from build123d import *

# Parameters (mm, degrees)
F3_DEPTH  = 6.86
F4_SIZE   = 0.13
F5_SIZE   = 0.06
F6_SIZE   = 0.03
F8_DEPTH  = 6.79
F10_DEPTH = 14.1


with BuildPart() as f1:
    # F0 (on Top) → F1 (revolve)
    with BuildSketch(Plane.XY):
        Polygon((-33.448007, 1.065), (-29.198007, 1.065), (-29.198007, 1.27955), (-29.778007, 1.27955), (-29.778007, 1.5), (-30.008007, 1.5), (-30.008007, 2.5), (-30.138007, 2.5), (-30.138007, 2.375), (-32.138007, 2.375), (-32.138007, 2.5), (-32.268007, 2.5), (-32.268007, 1.5), (-32.491007, 1.5), (-32.491007, 1.27955), (-33.111007, 1.27955), (-33.111007, 1.215), (-34.191007, 1.215), (-34.191007, 0), (-33.448007, 0), align=None)
    revolve(axis=Axis((-33.819507, 0, 0), (1, 0, 0)))

    # F2 (on face) → F3 (cut)
    with BuildSketch(Plane(origin=(-34.191007, 0, 0), x_dir=(0, -1, 0), z_dir=(-1, 0, 0))):
        with BuildLine():
            Line((-0.07875, 0.268), (-0.07875, 0.180575))
            ThreePointArc((-0.07875, 0.180575), (0, -0.197), (0.07875, 0.180575))
            Line((0.07875, 0.180575), (0.07875, 0.268))
            Line((0.07875, 0.268), (0, 0.268))
            Line((0, 0.268), (-0.07875, 0.268))
        make_face()
    extrude(amount=-F3_DEPTH, mode=Mode.SUBTRACT)

    # F4
    f4_edges = [f1.edges().sort_by_distance(p)[0] for p in [
        (-34.191007, -1.215, 0),
        (-32.491007, -1.5, 0),
        (-29.778007, -1.5, 0),
    ]]
    chamfer(f4_edges, length=F4_SIZE)

    # F5
    f5_edges = [f1.edges().sort_by_distance(p)[0] for p in [
        (-29.198007, -1.27955, 0),
    ]]
    chamfer(f5_edges, length=F5_SIZE)

    # F6
    f6_edges = [f1.edges().sort_by_distance(p)[0] for p in [
        (-33.111007, -1.27955, 0),
    ]]
    chamfer(f6_edges, length=F6_SIZE)

    # F7 (on face) → F8 (cut)
    with BuildSketch(Plane(origin=(-32.268007, 0, 0), x_dir=(0, -1, 0), z_dir=(-1, 0, 0))):
        with BuildLine():
            ThreePointArc((-0.503698, 1.550222), (0, 1.63), (0.503698, 1.550222))
            ThreePointArc((0.503698, 1.550222), (0.856518, 1.729993), (0.676747, 2.082814))
            ThreePointArc((0.676747, 2.082814), (0, 2.19), (-0.676747, 2.082814))
            ThreePointArc((-0.676747, 2.082814), (-0.856518, 1.729993), (-0.503698, 1.550222))
        make_face()
        with BuildLine():
            ThreePointArc((-1.594381, 0.338896), (-1.411621, 0.815), (-1.090683, 1.211326))
            ThreePointArc((-1.090683, 1.211326), (-1.069959, 1.606763), (-1.465396, 1.627487))
            ThreePointArc((-1.465396, 1.627487), (-1.896596, 1.095), (-2.142143, 0.455327))
            ThreePointArc((-2.142143, 0.455327), (-1.926477, 0.12323), (-1.594381, 0.338896))
        make_face()
        with BuildLine():
            ThreePointArc((-1.090683, -1.211326), (-1.411621, -0.815), (-1.594381, -0.338896))
            ThreePointArc((-1.594381, -0.338896), (-1.926477, -0.12323), (-2.142143, -0.455327))
            ThreePointArc((-2.142143, -0.455327), (-1.896596, -1.095), (-1.465396, -1.627487))
            ThreePointArc((-1.465396, -1.627487), (-1.069959, -1.606763), (-1.090683, -1.211326))
        make_face()
        with BuildLine():
            ThreePointArc((0.503698, -1.550222), (0, -1.63), (-0.503698, -1.550222))
            ThreePointArc((-0.503698, -1.550222), (-0.856518, -1.729993), (-0.676747, -2.082814))
            ThreePointArc((-0.676747, -2.082814), (0, -2.19), (0.676747, -2.082814))
            ThreePointArc((0.676747, -2.082814), (0.856518, -1.729993), (0.503698, -1.550222))
        make_face()
        with BuildLine():
            ThreePointArc((1.594381, -0.338896), (1.411621, -0.815), (1.090683, -1.211326))
            ThreePointArc((1.090683, -1.211326), (1.069959, -1.606763), (1.465396, -1.627487))
            ThreePointArc((1.465396, -1.627487), (1.896596, -1.095), (2.142143, -0.455327))
            ThreePointArc((2.142143, -0.455327), (1.926477, -0.12323), (1.594381, -0.338896))
        make_face()
        with BuildLine():
            ThreePointArc((1.090683, 1.211326), (1.411621, 0.815), (1.594381, 0.338896))
            ThreePointArc((1.594381, 0.338896), (1.926477, 0.12323), (2.142143, 0.455327))
            ThreePointArc((2.142143, 0.455327), (1.896596, 1.095), (1.465396, 1.627487))
            ThreePointArc((1.465396, 1.627487), (1.069959, 1.606763), (1.090683, 1.211326))
        make_face()
    extrude(amount=-F8_DEPTH, mode=Mode.SUBTRACT)

    # F9 (on face) → F10 (cut)
    with BuildSketch(Plane(origin=(-32.268007, 0, 0), x_dir=(0, -1, 0), z_dir=(-1, 0, 0))):
        with BuildLine():
            ThreePointArc((-1.594381, 0.338896), (-1.411621, 0.815), (-1.090683, 1.211326))
            ThreePointArc((-1.090683, 1.211326), (-1.069959, 1.606763), (-1.465396, 1.627487))
            ThreePointArc((-1.465396, 1.627487), (-1.896596, 1.095), (-2.142143, 0.455327))
            ThreePointArc((-2.142143, 0.455327), (-1.926477, 0.12323), (-1.594381, 0.338896))
        make_face()
        with BuildLine():
            ThreePointArc((-2.142143, -0.455327), (-1.896596, -1.095), (-1.465396, -1.627487))
            ThreePointArc((-1.465396, -1.627487), (-1.069959, -1.606763), (-1.090683, -1.211326))
            ThreePointArc((-1.090683, -1.211326), (-1.411621, -0.815), (-1.594381, -0.338896))
            ThreePointArc((-1.594381, -0.338896), (-1.926477, -0.12323), (-2.142143, -0.455327))
        make_face()
        with BuildLine():
            ThreePointArc((-0.676747, -2.082814), (0, -2.19), (0.676747, -2.082814))
            ThreePointArc((0.676747, -2.082814), (0.856518, -1.729993), (0.503698, -1.550222))
            ThreePointArc((0.503698, -1.550222), (0, -1.63), (-0.503698, -1.550222))
            ThreePointArc((-0.503698, -1.550222), (-0.856518, -1.729993), (-0.676747, -2.082814))
        make_face()
        with BuildLine():
            ThreePointArc((1.465396, -1.627487), (1.896596, -1.095), (2.142143, -0.455327))
            ThreePointArc((2.142143, -0.455327), (1.926477, -0.12323), (1.594381, -0.338896))
            ThreePointArc((1.594381, -0.338896), (1.411621, -0.815), (1.090683, -1.211326))
            ThreePointArc((1.090683, -1.211326), (1.069959, -1.606763), (1.465396, -1.627487))
        make_face()
        with BuildLine():
            ThreePointArc((2.142143, 0.455327), (1.896596, 1.095), (1.465396, 1.627487))
            ThreePointArc((1.465396, 1.627487), (1.069959, 1.606763), (1.090683, 1.211326))
            ThreePointArc((1.090683, 1.211326), (1.411621, 0.815), (1.594381, 0.338896))
            ThreePointArc((1.594381, 0.338896), (1.926477, 0.12323), (2.142143, 0.455327))
        make_face()
        with BuildLine():
            ThreePointArc((-0.503698, 1.550222), (0, 1.63), (0.503698, 1.550222))
            ThreePointArc((0.503698, 1.550222), (0.856518, 1.729993), (0.676747, 2.082814))
            ThreePointArc((0.676747, 2.082814), (0, 2.19), (-0.676747, 2.082814))
            ThreePointArc((-0.676747, 2.082814), (-0.856518, 1.729993), (-0.503698, 1.550222))
        make_face()
    extrude(amount=-F10_DEPTH, mode=Mode.SUBTRACT)


solid = f1.part
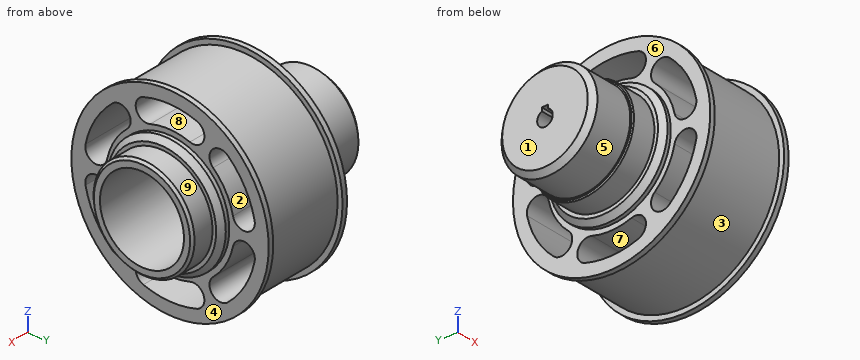
Could you check a few things on this model? Use its own coordinates, in mm. Face numbers are marked on the shaded views. A direction names the side the tool comes from. Give positions to 0.01 mm unless a question says otherwise; leave off trailing zeros. Loops run counter-clockwise (first coordinate to the right, second up) from the corner with the lowest first, then second, coordinate; pieces in that order, holes last. Notation, with made-up numbers: (54, 69.5) -> (83, 69.5) arc R31 cw to (83, 105.5) -> close; hole circle Ø10 at (24.5, -3.75). An arc over 180 degrees is marked (long way). Return JSON: item names as keys, results as strings.
Item 1: I'm going to push flat-ended pins straight in: pin 1 (2.5 mm diameter, centred on y = -1, z = -1, fed in from +X); pin 2 (1.7 mm diameter, centred on y = 0, z = 0, fed in from +X); pin 3 (2 mm diameter, centred on x = -30, z = -1.5, fed in from +Y). Where does each tip first touch, or does it pass through?
Geometry results:
{"pin 1": "stops at x = -29.2", "pin 2": "stops at x = -33.45", "pin 3": "stops at y = 2.45"}
Item 2: We'd pull the mould along Y, two halves only. Please class the marked faces 6, 7, 8 and 9: +Y half, -Y half, draft (parallel to the pull), parting line (faces both ways), or undercut.
Geometry results:
{"face 6": "draft", "face 7": "undercut", "face 8": "undercut", "face 9": "parting line"}
Item 3: If we section it at A-A on y = 1.8: List the corners of the cut face in (x, z) for me.
Geometry results:
{"outline": "(-32.27, -1.73) -> (-32.14, -1.73) -> (-32.14, -1.55) -> (-30.14, -1.55) -> (-30.14, -1.73) -> (-30.01, -1.73) -> (-30.01, -1.25) -> (-32.27, -1.25) -> close; (-32.27, -0.13) -> (-30.01, -0.13) -> (-30.01, 0.13) -> (-32.27, 0.13) -> close; (-32.27, 1.25) -> (-30.01, 1.25) -> (-30.01, 1.73) -> (-30.14, 1.73) -> (-30.14, 1.55) -> (-32.14, 1.55) -> (-32.14, 1.73) -> (-32.27, 1.73) -> close"}
Item 4: If we section it at B-B on x = -30.5: List the corners of the cut face in (y, z) for me (3 decimals), plus the area to 3 significant figures.
Geometry results:
{"outline": "circle Ø4.75 at (0, 0); hole (-2.142, -0.455) arc R2.19 ccw to (-1.465, -1.627) arc R0.28 ccw to (-1.091, -1.211) arc R1.63 cw to (-1.594, -0.339) arc R0.28 ccw to start; hole (-2.142, 0.455) arc R0.28 ccw to (-1.594, 0.339) arc R1.63 cw to (-1.091, 1.211) arc R0.28 ccw to (-1.465, 1.627) arc R2.19 ccw to start; hole circle Ø2.13 at (0, 0); hole (-0.677, -2.083) arc R2.19 ccw to (0.677, -2.083) arc R0.28 ccw to (0.504, -1.55) arc R1.63 cw to (-0.504, -1.55) arc R0.28 ccw to start; hole (-0.677, 2.083) arc R0.28 ccw to (-0.504, 1.55) arc R1.63 cw to (0.504, 1.55) arc R0.28 ccw to (0.677, 2.083) arc R2.19 ccw to start; hole (1.091, -1.211) arc R0.28 ccw to (1.465, -1.627) arc R2.19 ccw to (2.142, -0.455) arc R0.28 ccw to (1.594, -0.339) arc R1.63 cw to start; hole (1.091, 1.211) arc R1.63 cw to (1.594, 0.339) arc R0.28 ccw to (2.142, 0.455) arc R2.19 ccw to (1.465, 1.627) arc R0.28 ccw to start", "area": "8.65 mm²"}
Item 5: Which directions (+Z, -Z, +X, -X, +Y, -Y) give clear straight access to the entire face, cutting with the end or side of a thin tool? Please do the marked faces 1, 2, 3, 4 and 5.
Geometry results:
{"face 1": "+Z, -Z, -X, +Y, -Y", "face 2": "+X, -X", "face 3": "none", "face 4": "+X", "face 5": "-X"}
Item 6: If we section it at C-C on y = 0: Count the separate pieces of the cut face and the enclosed holes in it, plus the area to 3 significant figures.
Geometry results:
{"separate pieces": "4", "enclosed holes": "0", "area": "5.87 mm²"}
Item 7: I need wall thicknesses on L1, parallel to Z at x = -33.6, y = 0 (3 decimals); L2, parallel to Z at x = -32, y = 1.35; L3, parallel to Z at x = -31.85, y = 0.75. Which ranges of each line are inside material? Lowest first, please. Write a range as from..to.
Geometry results:
{"L1": "z = -1.215..-0.197, 0.268..1.215", "L2": "z = -1.95..-1.69, -0.91..0.91, 1.69..1.95", "L3": "z = -2.25..-2.05, -1.59..-0.76, 0.76..1.59, 2.05..2.25"}
